Work out the finished part from the listing and answer in its coordinate system (mm). A direction names the side the tool comes from. Coordinates: 2 decimals unless noted, no trailing zeros. Loops run counter-clockwise (first coordinate to the right, second up) from the corner with the lowest first, then second, coordinate; pieces in that order, holes last. Notation, with made-up numbers: (47, 52) - (72, 52) arc R17 ccw to (72, 67) - close; hole circle Ø11 at (62, 40.25). An arc over 180 degrees is marked (long way). Write each question's results on one line, items separated by ' | '. Start each with the question number.
1. A cutting plane is placed at A-A on z = 0. Determine the outline of the cut face in (x, y), then the cut area to 3 significant figures.
2. A cutting plane is placed at B-B on x = 67. Determine the outline of the cut face in (y, z).
3. Each of these flat-tipped pins is pushed along its axis until it touches: P1, Ø1, axis at y = 3, z = 23.5, coming from the +X side; P2, Ø1.5, axis at y = 3, z = -2, coming from the -X side. Where does it stop, or does it pass through?
4. Which of the six approach directions +Z, -Z, +X, -X, +Y, -Y give full straight-line access (tool end or side, diameter ignored) to faces 1 (the flat face through (74, 4.762, -21)), 2 (the flat face through (1.15, 2.35, -90.96))?
5. Find the intervals of material crossed by line 1 along Z through (x, y) = (-53, 4.4); line 2 along Z through (x, y) = (-42, 3.5); line 3 along X through (y, z) = (1.55, -20.5), in increasing order. Write a range as [from, to].
6. Determine the mould class of faces 3 (the flat face through (74, 0, -21)), 4 (the cylindrical face through (-14.468, 2.348, 91.165)), 5 (the flat face through (-1.15, 2.35, 90.96)) for opening direction Z: released by +Z, released by -Z, zero draft, split by the parting line, or undercut.
Autodesk Inventor part; units mm, degrees
ref_plane "YZ Plane" through (0, 0, 0) normal (1, 0, 0) x (0, 1, 0)
ref_plane "XZ Plane" through (0, 0, 0) normal (0, 1, 0) x (-1, 0, 0)
ref_plane "XY Plane" through (0, 0, 0) normal (0, 0, 1) x (1, 0, 0)
sketch "Sketch1" plane through (0, 0, 0) normal (0, 1, 0) x (-1, 0, 0)
  circle A0 centre (0, 0) radius 76.2
  circle A1 centre (0, 0) radius 82.55
  line L0 (0, 0) -> (0, -82.55) construction
  line L1 (0, -95.25) -> (-3.422, -82.479)
  arc A2 (-25.4, -78.5452) -> (0, -95.25) centre (0, -67.587) ccw
  line L2 (0, 95.25) -> (3.422, 82.479)
  arc A3 (25.4, 78.5452) -> (0, 95.25) centre (0, 67.587) ccw
  point P0 (0, 82.55)
  point P1 (25.4, 78.5452)
  dimension "d0" = 152.4
  dimension "d1" = 6.35
  dimension "d4" = 15
  dimension "d5" = 12.7
  dimension "d6" = 25.4
  dimension "d9" = 360
extrude "Extrusion1" add sketch "Sketch1" along normal blind 4.7625
fillet "Fillet1" radius 3.175 4 edges at (25.4, 2.3813, -78.5452) (3.422, 2.3813, -82.479) (-25.4, 2.3813, 78.5452) (-3.422, 2.3813, 82.479)
sketch "Sketch2" plane through (0, 4.7625, 0) normal (0, 1, 0) x (1, 0, 0)
  line L0 (0, 95.25) -> (2.3329, 86.5436)
  circle A0 centre (0, 0) radius 95.25 construction
properties part number "Blade - Ring" material "Steel, Mild"
Values:
1) outline: (-82.55, 0) - (-76.2, 0) - (-76.2, 4.76) - (-82.55, 4.76) - close; (76.2, 0) - (82.55, 0) - (82.55, 4.76) - (76.2, 4.76) - close | area: 60.5 mm^2
2) outline: (0, -48.22) - (4.76, -48.22) - (4.76, -36.3) - (0, -36.3) - close; (0, 36.3) - (4.76, 36.3) - (4.76, 48.22) - (0, 48.22) - close
3) P1: x = 79.28 | P2: x = -82.54
4) face 1: +Z, -Z, +X, -X, +Y | face 2: -X, +Y, -Y
5) line 1: [-63.29, -54.75], [54.75, 63.29] | line 2: [-71.07, -63.58], [63.58, 71.07] | line 3: [-79.96, -73.39], [73.39, 79.96]
6) face 3: zero draft | face 4: released by +Z | face 5: undercut
